For this review, take the finished solid that the model builds, in its own axes (mm). A direction names the side the tool comes from. Give positions to 0.01 mm unless a question says otherwise; leave off trailing zeros. Order: outer loops, then holes, each group sorted by start corner. A loop starts at its lowest first (then second) coordinate and runs counter-clockwise, first axis right, second up. Notation, with made-up numbers: (85, -35) -> (129, -35) arc R15 ccw to (129, -12) -> close; hole circle Ø6 at (-24.5, 50.5). An arc over 180 degrees is marked (long way). One line per item, written item: value. Start each with the question number.
Autodesk Inventor part; units mm, degrees
ref_plane "YZ Plane" through (0, 0, 0) normal (1, 0, 0) x (0, 1, 0)
ref_plane "XZ Plane" through (0, 0, 0) normal (0, 1, 0) x (-1, 0, 0)
ref_plane "XY Plane" through (0, 0, 0) normal (0, 0, 1) x (1, 0, 0)
sketch "Sketch1" plane through (0, 0, 0) normal (1, 0, 0) x (0, 1, 0)
  line L0 (30.48, -20.9755) -> (30.48, 20.9755)
  line L1 (-30.48, 20.9755) -> (-30.48, -20.9755)
  arc A0 (30.48, 20.9755) -> (-30.48, 20.9755) centre (0, 0) ccw
  arc A1 (-30.48, -20.9755) -> (30.48, -20.9755) centre (0, 0) ccw
  arc A2 (-30.48, -46.9784) -> (-30.48, 46.9784) centre (0, 0) ccw
  line L2 (-60.48, 32) -> (-60.48, -32)
  arc A3 (-60.48, 32) -> (-30.48, 46.9784) centre (-111.7897, 172.2999) ccw
  arc A4 (-30.48, -46.9784) -> (-60.48, -32) centre (-111.7897, -172.2999) ccw
  line L3 (56, 0) -> (0, 0) construction
  line L4 (0, 0) -> (-28, 48.4974) construction
  line L5 (0, 0) -> (-28, -48.4974) construction
  line L6 (30.48, 0) -> (56, 0) construction
  line L7 (-18.5, -32.0429) -> (-28, -48.4974) construction
  line L8 (-28, 48.4974) -> (-18.5, 32.0429) construction
  circle A5 centre (43.24, 0) radius 4.5
  circle A6 centre (-23.25, -40.2702) radius 4.5
  circle A7 centre (-23.25, 40.2702) radius 4.5
  point P0 (-60.48, 0)
  point P1 (-30.48, 0)
  dimension "d1" = 60.96
  dimension "d2" = 30.48
  dimension "d3" = 37
  dimension "d4" = 37
  dimension "d5" = 19
  dimension "d6" = 64
  dimension "d7" = 120
  dimension "d8" = 120
  dimension "d9" = 9
  dimension "d10" = 9
  dimension "d11" = 9
  dimension "d14" = 30
extrude "Extrusion1" add sketch "Sketch1" along normal blind 3
properties part number "battlebotmotorbracetemp"
Q1. Take a section at A-A (y = 0). State the section outline as (x, z) points, and give its area (3 significant figures).
Q2. Take a section at D-D (y = -23.25). State the section outline as (x, z) points.
Q3. For faces 5 (the flat face through (1, 30.48, 0)), 6 (the flat face through (0, -29, 26)), list the 3-axis set-ups (+Z, -Z, +X, -X, +Y, -Y) from which the entire face can be reached by the end or side of a thin tool; tool diameter is ignored.
Q4. For line 1 along Z through (x, y) = (2.1, -23.25); line 2 along Y through (x, z) = (2.1, -23.5); line 3 along Y through (x, z) = (2.3, 13.5), list the stretches that pass through material, from the lowest coordinate up.
Q5. Take a section at B-B (z = 0). State the section outline as (x, y) points, and give its area (3 significant figures).
Q6. Take a section at C-C (x = 1.65). State the section outline as (y, z) points.
Q7. For pin 1 Ø1.5 at (x, z) = (1.5, 9.5) entering from +Y; pin 2 Ø1.5 at (x, y) = (2, 19.5) entering from +Z; pin 3 Ø1 at (x, y) = (0.5, 30) entering from +Z, all flat-tipped, find the tip position at first contact; note any pin that passes through.
Q8. Mouldability with a two-part tool opening along Z and no side actions: class faces 1 (the cylindrical face through (1.479, 47.532, -1.352)), 2 (the cylindrical face through (1.48, -45.27, -38.54)), 3 (the flat face through (3, -29, 26)), 4 (the flat face through (1, -30.48, 0)) as pulls with the +Z half, pulls with the -Z half, needs draft (parallel to the pull), parting line crosses it, or undercut.
Answers below:
1. outline: (0, -56) -> (3, -56) -> (3, -37) -> (0, -37) -> close; (0, 37) -> (3, 37) -> (3, 56) -> (0, 56) -> close
1. area: 114 mm²
2. outline: (0, -50.95) -> (3, -50.95) -> (3, -44.77) -> (0, -44.77) -> close; (0, -35.77) -> (3, -35.77) -> (3, -28.78) -> (0, -28.78) -> close; (0, 28.78) -> (3, 28.78) -> (3, 35.77) -> (0, 35.77) -> close; (0, 44.77) -> (3, 44.77) -> (3, 50.95) -> (0, 50.95) -> close
3. face 5: +X, -X
3. face 6: +Z, -Z, -X, +Y, -Y
4. line 1: z = -50.95 to -44.77, -35.77 to -28.78, 28.78 to 35.77, 44.77 to 50.95
4. line 2: y = -60.48 to -28.58, 28.58 to 50.83
4. line 3: y = -60.48 to -30.48, 30.48 to 54.35
5. outline: (0, -60.48) -> (3, -60.48) -> (3, -30.48) -> (0, -30.48) -> close; (0, 30.48) -> (3, 30.48) -> (3, 38.74) -> (0, 38.74) -> close; (0, 47.74) -> (3, 47.74) -> (3, 56) -> (0, 56) -> close
5. area: 140 mm²
6. outline: (-60.48, -32) arc R149.39 cw to (-30.48, -46.98) arc R56 ccw (long way) to (-30.48, 46.98) arc R149.39 cw to (-60.48, 32) -> close; hole (-30.48, -20.98) arc R37 ccw to (30.48, -20.98) -> (30.48, 20.98) arc R37 ccw to (-30.48, 20.98) -> close; hole circle Ø9 at (-23.25, -40.27); hole circle Ø9 at (-23.25, 40.27); hole circle Ø9 at (43.24, 0)
7. pin 1: stops at y = 55.31
7. pin 2: stops at z = 52.77
7. pin 3: stops at z = 47.6
8. face 1: undercut
8. face 2: pulls with the -Z half
8. face 3: needs draft
8. face 4: undercut
